from build123d import *

# Parameters (mm, degrees)
F2_R          = 1.27
F3_DEPTH      = 7.8750001
F3_DEPTH_BACK = 7.8750001
F5_D          = 4
F5_DEPTH      = 7.62
F5_TIP        = 1.2017212381


with BuildPart() as f1:
    # F0 (on Front) → F1 (revolve)
    with BuildSketch(Plane.XZ):
        with BuildLine():
            Line((0, 13.97), (0, 0))
            Line((0, 0), (6.985, 0))
            ThreePointArc((6.985, 0), (7.874, 0.889), (6.985, 1.778))
            add(Edge.make_bspline(
                [(0, 13.97), (1.6814160792, 13.8530222035), (4.2417061309, 10.8131539294), (5.8432030034, 7.0071502602), (6.7403060068, 3.5219468301), (6.985, 1.778)],
                knots=[0, 0, 0, 0, 0.3381752407, 0.6530157142, 1, 1, 1, 1], degree=3))
        make_face()
    revolve(axis=Axis((0, 0, 11.4008450556), (0, 0, 1)))

    # F2 (on Front) → F3 (cut, two sides)
    with BuildSketch(Plane.XZ) as f3_sk:
        with Locations((0, 10.16)):
            Circle(F2_R)
    extrude(amount=-F3_DEPTH, mode=Mode.SUBTRACT)
    extrude(f3_sk.sketch, amount=F3_DEPTH_BACK, mode=Mode.SUBTRACT)

    # F5
    with Locations(Plane(origin=(0, 0, 0), x_dir=(1, 0, 0), z_dir=(0, 0, -1))):
        with Locations((0, 0)):
            Hole(F5_D / 2, depth=F5_DEPTH)
            with Locations((0, 0, -(F5_DEPTH + F5_TIP / 2))):  # 118° drill point
                Cone(0, F5_D / 2, F5_TIP, mode=Mode.SUBTRACT)


solid = f1.part
The listing builds one solid part. Answer for the finished solid, in the listing's coordinates (mm). Coordinates: 2 decimals unless noted, no trailing zeros.
Q1. Given P1, Ø3, axis at x = -2, z = 6.5, coming from the -Y side; P2, Ø2, axis at y = -1.5, z = 4.5, coming from the -X side; P3, Ø4, axis at y = -0.5, z = 10, coming from the -X side; P4, Ø6.5, axis at x = 0, y = 0, coming from the -Z side, each flat-ended and moving along its own axis, determine where each tip first touches the part or whether it passes through.
Q2. Consider line 1 (Z direction, x = 0, y = 1.25); line 2 (Y direction, x = 0.75, z = 3.5); line 3 (Y direction, x = -1.75, z = 4.25). Determine where each line is inside the solid, lowest interval first.
Q3. For a pull along Z with two mould halves and no side action, classify faces 1 (the face through (-0.28, -0.07, 8.92)), 2 (the face through (-0.08, 0.34, 8.61)), 3 (the face through (0, 2, 4)) as pulls with the +Z half, pulls with the -Z half, needs draft (parallel to the pull), parting line crosses it, or undercut.
Answers follow:
1. P1: stops at y = -6.14
1. P2: stops at x = -6.58
1. P3: stops at x = -5.36
1. P4: stops at z = 0
2. line 1: z = 8.07 to 8.89, 11.43 to 13.61
2. line 2: y = -6.64 to -1.85, 1.85 to 6.64
2. line 3: y = -6.27 to -0.97, 0.97 to 6.27
3. face 1: undercut
3. face 2: pulls with the -Z half
3. face 3: needs draft
